from build123d import *

# Parameters (mm, degrees)
SKETCH_2_R          = 14
CUT_EXTRUDE_1_DEPTH = 20
SKETCH_3_R          = 30
EXTRUDE_1_DEPTH     = 20
SKETCH_4_R          = 12.5
EXTRUDE_2_DEPTH     = 5
CHAMFER_1_SIZE      = 1
SKETCH_5_R          = 3
CUT_EXTRUDE_2_DEPTH = 15


with BuildPart() as part:
    # 草图1 → 旋转1 (revolve)
    with BuildSketch(Plane.XY):
        Polygon((0, 0), (0, 15), (-70, 15), (-70, 5), (-85, 5), (-85, 0), align=None)
    revolve(axis=Axis((0, 0, 0), (0, 1, 0)))

    # 草图2 → 切除-拉伸1 (cut)
    with BuildSketch(Plane(origin=(0, 0, 0), x_dir=(1, 0, 0), z_dir=(0, 1, 0))):
        with Locations((50, 0)):
            Circle(SKETCH_2_R)
    extrude(amount=CUT_EXTRUDE_1_DEPTH, mode=Mode.SUBTRACT)

    # 草图3 → 凸台-拉伸1 (add)
    with BuildSketch(Plane(origin=(0, 15, 0), x_dir=(1, 0, 0), z_dir=(0, 1, 0))):
        Circle(SKETCH_3_R)
    extrude(amount=EXTRUDE_1_DEPTH)

    # 草图4 → 凸台-拉伸2 (add)
    with BuildSketch(Plane(origin=(0, 35, 0), x_dir=(1, 0, 0), z_dir=(0, 1, 0))):
        Circle(SKETCH_4_R)
    extrude(amount=EXTRUDE_2_DEPTH)

    # 倒角1
    chamfer_1_edges = [part.edges().sort_by_distance(p)[0] for p in [
        (-12.5, 40, 0),
    ]]
    chamfer(chamfer_1_edges, length=CHAMFER_1_SIZE)

    # 草图5 → 切除-拉伸2 (cut)
    with BuildSketch(Plane(origin=(0, 35, 0), x_dir=(1, 0, 0), z_dir=(0, 1, 0))):
        with Locations((0, 20)):
            Circle(SKETCH_5_R)
        with Locations((17.320508076, -10)):
            Circle(SKETCH_5_R)
        with Locations((-17.320508076, -10)):
            Circle(SKETCH_5_R)
    extrude(amount=-CUT_EXTRUDE_2_DEPTH, mode=Mode.SUBTRACT)


solid = part.part
Verification items for the finished model (mm, model axes). A direction names the side the tool comes from. Round coordinates to 2 decimals unless told otherwise and drop trailing zeros. Loops run counter-clockwise (first coordinate to the right, second up) from the corner with the lowest first, then second, coordinate; pieces in that order, holes last. Notation, with made-up numbers: (77, 5.5) - (130, 5.5) arc R25 cw to (130, 36.5) - close; hole circle Ø6 at (-37.75, -11.75). An arc over 180 degrees is marked (long way). Answer in a Markdown table with one row per item. Add a question column.
Q1. Release check for a two-part mould opening along X. For faces 3 (the face through (-15.71, 27.6, 7.47)), 4 (the face through (-0.65, 27.6, -17.07)), 5 (the face through (0, 35, 13)), 6 (the face through (11.923, 36.972, -3.755)) record: pulls with the +X half, pulls with the -X half, needs draft (parallel to the pull), parting line crosses it, or undercut.
Q2. Section check D-D on x = 50. Enter the section's corners in (y, z), plus the area to 3 significant figures.
Q3. Section check C-C on y = 24. Enter the section's corners in (x, z), plus the area to 3 significant figures.
Q4. Gauge pin test, flat ends, axial feed: pin 1 (1 mm diameter, centred on x = -22.5, z = -48.5, fed in from +Y); pin 2 (6 mm diameter, centred on y = 14, z = -19, fed in from +X); pin 3 (6.5 mm diameter, centred on x = -1.5, z = -21, fed in from +Y); pin 4 (9.5 mm diameter, centred on x = 0, z = -20, fed in from -Y). Record the tip position at first contact, or that the pin passes through.
Q5. Section check B-B on x = 0. Enter the section's corners in (y, z), plus the area to 3 significant figures.
Q6. Section check A-A on z = 0. Enter the section's corners in (x, y), plus the area to 3 significant figures.
Q7. Material ranges on line 1 (X direction, y = 29, z = 10); line 2 (Y direction, x = -51.5, z = -21.5); line 3 (Y direction, x = -12, z = -22), recorded low to high.
Q8. Tool access check on faces 1 (the face through (17, 20, 10)), 2 (the face through (67.453, 2.465, -51.721)). Record the directions out of +Z, -Z, +X, -X, +Y, -Y that give a thin tool (end or side, any length) a straight path to the whole face; none if there is none.
Found:
| question | item | result |
|---|---|---|
| 1 | face 3 | undercut |
| 1 | face 4 | undercut |
| 1 | face 5 | needs draft |
| 1 | face 6 | parting line crosses it |
| 2 | outline | (0, -68.74) - (5, -68.74) - (5, -48.99) - (15, -48.99) - (15, -14) - (0, -14) - close; (0, 14) - (15, 14) - (15, 48.99) - (5, 48.99) - (5, 68.74) - (0, 68.74) - close |
| 2 | area | 1,250 mm² |
| 3 | outline | circle Ø60 at (0, 0); hole circle Ø6 at (-17.32, 10); hole circle Ø6 at (0, -20); hole circle Ø6 at (17.32, 10) |
| 3 | area | 2,740 mm² |
| 4 | pin 1 | stops at y = 15 |
| 4 | pin 2 | stops at x = 68.15 |
| 4 | pin 3 | stops at y = 35 |
| 4 | pin 4 | stops at y = 0 |
| 5 | outline | (0, -85) - (5, -85) - (5, -70) - (15, -70) - (15, -30) - (35, -30) - (35, -23) - (20, -23) - (20, -17) - (35, -17) - (35, -12.5) - (39, -12.5) - (40, -11.5) - (40, 11.5) - (39, 12.5) - (35, 12.5) - (35, 30) - (15, 30) - (15, 70) - (5, 70) - (5, 85) - (0, 85) - close |
| 5 | area | 3,480 mm² |
| 6 | outline | (-85, 0) - (36, 0) - (36, 15) - (30, 15) - (30, 35) - (12.5, 35) - (12.5, 39) - (11.5, 40) - (-11.5, 40) - (-12.5, 39) - (-12.5, 35) - (-30, 35) - (-30, 15) - (-70, 15) - (-70, 5) - (-85, 5) - close; (64, 0) - (85, 0) - (85, 5) - (70, 5) - (70, 15) - (64, 15) - close |
| 6 | area | 3,150 mm² |
| 7 | line 1 | x = -28.28 to -20.32, -14.32 to 14.32, 20.32 to 28.28 |
| 7 | line 2 | y = 0 to 15 |
| 7 | line 3 | y = 0 to 35 |
| 8 | face 1 | +Y |
| 8 | face 2 | +Y, -Y |
